Part model, mm, in its own coordinate system. Face numbers are marked on the shaded views. A direction names the side the tool comes from. Round coordinates to 2 decimals unless told otherwise and drop trailing zeros. Write each loop counter-clockwise with the first axis right and the second up, starting at its lowest first coordinate (ties: lowest second). Pieces come first, ordered by that corner, then holes. Notation, with made-up numbers: (78, 43.25) -> (128, 43.25) arc R26 cw to (128, 78.25) -> close; hole circle Ø1 at (13, 79). An arc over 180 degrees is marked (long way). Return JSON: item names as keys, results as strings. Group by question number.
(1) Saw through at B-B (y = -29.5). List the corners of the cut face in (x, z), plus the area to 3 significant figures.
(2) Tool access for the marked faces 4 and 5: list every direction of +Z, -Z, +X, -X, +Y, -Y with a clear straight run to the whole face (end or side of a thin tool).
(3) Saw through at C-C (z = 58). List the corners of the cut face in (x, y).
(4) Drill centre lines: L1, parallel to Y at x = 152, z = 7; L2, parallel to Z at x = 108, y = -45; L3, parallel to X at y = -78, z = 62. Where is each one in solid material? Low to high. Write a range as from..to.
(5) Saw through at D-D (x = -3). List the corners of the cut face in (y, z) (3 decimals).
(6) Mould opens along Y. For the marked faces 1, 2 and 3 say: +Y half, -Y half, draft (parallel to the pull), parting line (faces both ways), or undercut.
(7) Saw through at A-A (x = 152.4). List the corners of the cut face in (y, z).
from build123d import *

# Parameters (mm, degrees)
F0_W     = 190.5
F0_H     = 12.7
F1_DEPTH = 82.55
F2_W     = 25.4
F2_H     = 127
F3_DEPTH = 82.55
F5_DEPTH = 25.401
F6_R     = 17.487125
F7_DEPTH = 25.401
F8_R     = 17.4625
F9_DEPTH = 25.4


with BuildPart() as f1:
    # F0 (on Front) → F1 (new body)
    with BuildSketch(Plane.XZ):
        with Locations((95.25, 6.35)):
            Rectangle(F0_W, F0_H)
    extrude(amount=F1_DEPTH)

    # F2 (on face) → F3 (join)
    with BuildSketch(Plane.XZ.offset(82.55)):
        with Locations((-12.7, 63.5)):
            Rectangle(F2_W, F2_H)
    extrude(amount=-F3_DEPTH)

    # F4 (on face) → F5 (cut, through all)
    with BuildSketch(Plane.YZ):
        with BuildLine():
            ThreePointArc((-82.55, 69.85), (-41.275, 111.125), (0, 69.85))
            Line((0, 69.85), (0, 127))
            Line((0, 127), (-82.55, 127))
            Line((-82.55, 127), (-82.55, 69.85))
        make_face()
    extrude(amount=-F5_DEPTH, mode=Mode.SUBTRACT)

    # F6 (on face) → F7 (cut, through all)
    with BuildSketch(Plane.YZ):
        with Locations((-41.275, 69.85)):
            Circle(F6_R)
    extrude(amount=-F7_DEPTH, mode=Mode.SUBTRACT)

    # F8 (on face) → F9 (cut)
    with BuildSketch(Plane.XY.offset(12.7)):
        with Locations((76.2, -41.275)):
            Circle(F8_R)
        with Locations((152.4, -41.275)):
            Circle(F8_R)
    extrude(amount=-F9_DEPTH, mode=Mode.SUBTRACT)


solid = f1.part
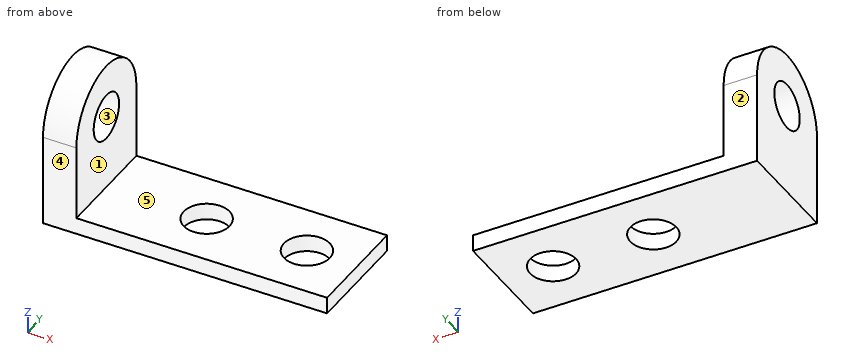
Computed values:
{
 "1": {"outline": "(-25.4, 0) -> (63.3, 0) -> (63.3, 12.7) -> (0, 12.7) -> (0, 56.92) -> (-25.4, 56.92) -> close; (-25.4, 82.78) -> (0, 82.78) -> (0, 109.41) -> (-25.4, 109.41) -> close; (89.1, 0) -> (139.5, 0) -> (139.5, 12.7) -> (89.1, 12.7) -> close; (165.3, 0) -> (190.5, 0) -> (190.5, 12.7) -> (165.3, 12.7) -> close", "area": "3,890 mm2"},
 "2": {"face 4": "+Z, -Z, +X, -X, -Y", "face 5": "+Z, +X, +Y, -Y"},
 "3": {"outline": "(-25.4, -82.55) -> (0, -82.55) -> (0, -54.13) -> (-25.4, -54.13) -> close; (-25.4, -28.42) -> (0, -28.42) -> (0, 0) -> (-25.4, 0) -> close"},
 "4": {"L1": "-82.55..-58.73, -23.82..0", "L2": "0..12.7", "L3": "-25.4..0"},
 "5": {"outline": "(-82.55, 0) -> (0, 0) -> (0, 69.85) arc R41.275 ccw to (-82.55, 69.85) -> close; hole circle Ø34.974 at (-41.275, 69.85)"},
 "6": {"face 1": "draft", "face 2": "+Y half", "face 3": "undercut"},
 "7": {"outline": "(-82.55, 0) -> (-58.74, 0) -> (-58.74, 12.7) -> (-82.55, 12.7) -> close; (-23.81, 0) -> (0, 0) -> (0, 12.7) -> (-23.81, 12.7) -> close"}
}
